Answer from the drawing. Dimensions are ordinates in mm from the lowest x, y and z of the part. Give positions to 0.01 mm unless a question says otherwise; leave off trailing zeros. Order: outer loops, then holes, each group sorted by start corner. A loop starts at its lowest first (then second) coordinate and runs counter-clockwise, first axis right, second up. Notation, with made-up numbers: (47, 42.25) -> (97, 42.25) arc R13 cw to (97, 53.25) -> close; hole circle Ø10 at (12, 61). An arc over 180 degrees is marked (long way). Answer as a JSON object with one key per item and string values. Group by question number.
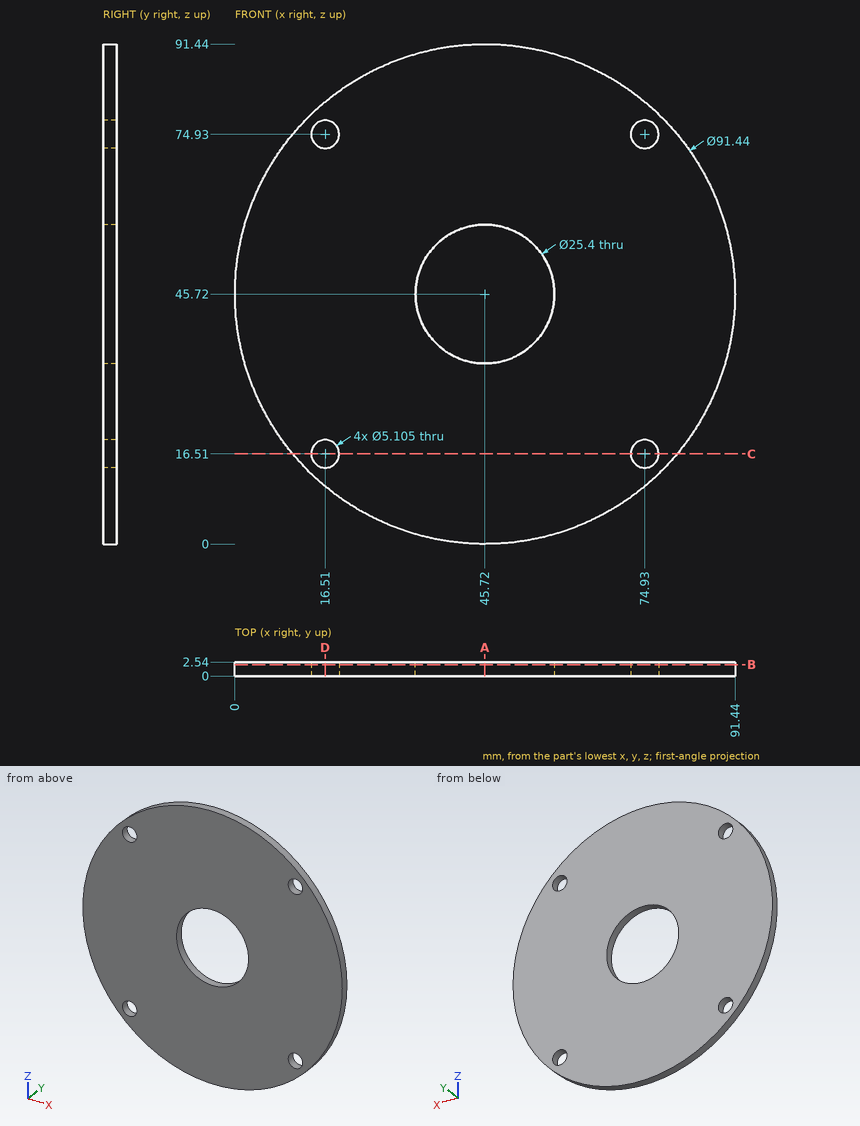
(1) Find the intervals of material crossed by line 1 along Z through (x, y) = (46, 1.55); line 2 along X through (y, z) = (0.25, 76.5) (1 decimal), in increasing order. Write a range as [from, to].
(2) A cutting plane is placed at D-D (x = 16.51). Determine the outline of the cut face in (y, z), and give its area (3 significant figures).
(3) A cutting plane is placed at C-C (z = 16.51). Determine the outline of the cut face in (x, y).
(4) A cutting plane is placed at A-A (x = 45.72). Determine the outline of the cut face in (y, z), and give its area (3 significant figures).
(5) A cutting plane is placed at B-B (y = 2.1). Determine the outline of the cut face in (x, z) (1 decimal).
Check sheet entries:
{
 "1": {"line 1": "z = [0, 33.02], [58.42, 91.44]", "line 2": "x = [11.9, 14.5], [18.5, 72.9], [76.9, 79.5]"},
 "2": {"outline": "(0, 10.55) -> (2.54, 10.55) -> (2.54, 13.96) -> (0, 13.96) -> close; (0, 19.06) -> (2.54, 19.06) -> (2.54, 72.38) -> (0, 72.38) -> close; (0, 77.48) -> (2.54, 77.48) -> (2.54, 80.89) -> (0, 80.89) -> close", "area": "153 mm2"},
 "3": {"outline": "(10.55, 0) -> (13.96, 0) -> (13.96, 2.54) -> (10.55, 2.54) -> close; (19.06, 0) -> (72.38, 0) -> (72.38, 2.54) -> (19.06, 2.54) -> close; (77.48, 0) -> (80.89, 0) -> (80.89, 2.54) -> (77.48, 2.54) -> close"},
 "4": {"outline": "(0, 0) -> (2.54, 0) -> (2.54, 33.02) -> (0, 33.02) -> close; (0, 58.42) -> (2.54, 58.42) -> (2.54, 91.44) -> (0, 91.44) -> close", "area": "168 mm2"},
 "5": {"outline": "circle Ø91.4 at (45.7, 45.7); hole circle Ø5.1 at (16.5, 16.5); hole circle Ø5.1 at (16.5, 74.9); hole circle Ø25.4 at (45.7, 45.7); hole circle Ø5.1 at (74.9, 16.5); hole circle Ø5.1 at (74.9, 74.9)"}
}
